Work out the finished part from the listing and answer in its coordinate system (mm). A direction names the side the tool comes from. Coordinates: 2 decimals unless noted, no trailing zeros. Loops run counter-clockwise (first coordinate to the right, second up) from the corner with the lowest first, then second, coordinate; pieces in that order, holes last. Notation, with made-up numbers: (17.5, 20.25) -> (61.5, 20.25) arc R9 ccw to (61.5, 29.25) -> close; hole circle Ø11 at (68, 60). An arc over 180 degrees is marked (long way). Use a Markdown table: item, result.
from build123d import *

# Parameters (mm, degrees)
EXTRUDE_1_DEPTH     = 2
SKETCH_2_R          = 1.6
CUT_EXTRUDE_1_DEPTH = 3
SKETCH_3_W          = 3
SKETCH_3_H          = 24
SKETCH_3_W_2        = 4
CUT_EXTRUDE_2_DEPTH = 3
SKETCH_4_W          = 10
SKETCH_4_H          = 2
EXTRUDE_2_DEPTH     = 2
SKETCH_5_R          = 0.5
CUT_EXTRUDE_3_DEPTH = 2
SKETCH_6_R          = 0.5
CUT_EXTRUDE_4_DEPTH = 2


with BuildPart() as part:
    # 草图1 → 凸台-拉伸1 (new body)
    with BuildSketch(Plane.XY):
        Polygon((0, 0), (17, 0), (17, 2.5), (20, 2.5), (20, 14.5), (17, 14.5), (17, 51.5), (0, 51.5), align=None)
    extrude(amount=EXTRUDE_1_DEPTH)

    # 草图2 → 切除-拉伸1 (cut, through all)
    with BuildSketch(Plane.XY.offset(2)):
        with Locations((9, 5.5)):
            Circle(SKETCH_2_R)
        with Locations((9, 16.5)):
            Circle(SKETCH_2_R)
    extrude(amount=-CUT_EXTRUDE_1_DEPTH, mode=Mode.SUBTRACT)

    # 草图3 → 切除-拉伸2 (cut, through all)
    with BuildSketch(Plane.XY.offset(2)):
        with Locations((15.5, 39.5)):
            Rectangle(SKETCH_3_W, SKETCH_3_H)
        with Locations((2, 39.5)):
            Rectangle(SKETCH_3_W_2, SKETCH_3_H)
    extrude(amount=-CUT_EXTRUDE_2_DEPTH, mode=Mode.SUBTRACT)

    # 草图4 → 凸台-拉伸2 (add)
    with BuildSketch(Plane(origin=(0, 51.5, 0), x_dir=(1, 0, 0), z_dir=(0, 1, 0))):
        with Locations((9, -1)):
            Rectangle(SKETCH_4_W, SKETCH_4_H)
    extrude(amount=EXTRUDE_2_DEPTH)

    # 草图5 → 切除-拉伸3 (cut)
    with BuildSketch(Plane(origin=(0, 0, 0), x_dir=(-1, 0, 0), z_dir=(0, 0, -1))):
        with Locations((-14, 27.5)):
            Circle(SKETCH_5_R)
        with Locations((-4, 27.5)):
            Circle(SKETCH_5_R)
    extrude(amount=-CUT_EXTRUDE_3_DEPTH, mode=Mode.SUBTRACT)

    # 草图6 → 切除-拉伸4 (cut)
    with BuildSketch(Plane(origin=(0, 0, 0), x_dir=(-1, 0, 0), z_dir=(0, 0, -1))):
        with Locations((-17, 14.5)):
            Circle(SKETCH_6_R)
        with Locations((-17, 2.5)):
            Circle(SKETCH_6_R)
    extrude(amount=-CUT_EXTRUDE_4_DEPTH, mode=Mode.SUBTRACT)


solid = part.part
Q1. Section B-B on y = 5.5 is taken. Determine the outline of the cut face in (x, z).
Solved:
| item | result |
|---|---|
| outline | (0, 0) -> (7.4, 0) -> (7.4, 2) -> (0, 2) -> close; (10.6, 0) -> (20, 0) -> (20, 2) -> (10.6, 2) -> close |
Q2. Given pin 1 Ø3.5 at (x, y) = (9, 5.5) entering from +Z; pin 2 Ø1 at (y, z) = (24, 1.5) entering from +X; pin 3 Ø0.6 at (x, z) = (1, 1) entering from +Y; pin 4 Ø1 at (y, z) = (39.5, 1) entering from +X, each flat-ended and moving along its own axis, determine where each tip first touches the part or whether it passes through.
Solved:
| item | result |
|---|---|
| pin 1 | z = 2 |
| pin 2 | x = 17 |
| pin 3 | y = 27.5 |
| pin 4 | x = 14 |
Q3. Section C-C on x = 2.25 is taken. Determine the outline of the cut face in (y, z).
Solved:
| item | result |
|---|---|
| outline | (0, 0) -> (27.5, 0) -> (27.5, 2) -> (0, 2) -> close |
Q4. Consider line 1 (Y direction, x = 9, z = 0.65); line 2 (X direction, y = 25.5, z = 0.1); line 3 (Y direction, x = 15.5, z = 1.35). Determine where each line is inside the solid, lowest interval first. Write a range as [from, to].
Solved:
| item | result |
|---|---|
| line 1 | [0, 3.9], [7.1, 14.9], [18.1, 53.5] |
| line 2 | [0, 17] |
| line 3 | [0, 27.5] |
Q5. Determine the mould class of faces 4 (the cylindrical face through (17, 14, 1)), 5 (the flat face through (14, 41, 1)), 6 (the flat face through (8, 0, 1)), 7 (the flat face through (0, 14, 1)) for opening direction X: pulls with the +X half, pulls with the -X half, needs draft (parallel to the pull), parting line crosses it, or undercut.
Solved:
| item | result |
|---|---|
| face 4 | undercut |
| face 5 | pulls with the +X half |
| face 6 | needs draft |
| face 7 | pulls with the -X half |
Q6. Section A-A on z = 1 is taken. Determine the outline of the cut face in (x, y), and give its area (3 significant figures).
Solved:
| item | result |
|---|---|
| outline | (0, 0) -> (17, 0) -> (17, 2) arc R0.5 cw (long way) to (17.5, 2.5) -> (20, 2.5) -> (20, 14.5) -> (17.5, 14.5) arc R0.5 cw (long way) to (17, 15) -> (17, 27.5) -> (14.5, 27.5) arc R0.5 cw (long way) to (14, 28) -> (14, 53.5) -> (4, 53.5) -> (4, 28) arc R0.5 cw (long way) to (3.5, 27.5) -> (0, 27.5) -> close; hole circle Ø3.2 at (9, 5.5); hole circle Ø3.2 at (9, 16.5) |
| area | 745 mm² |
Q7. Section D-D on y = 29 is taken. Determine the outline of the cut face in (x, z).
Solved:
| item | result |
|---|---|
| outline | (4, 0) -> (14, 0) -> (14, 2) -> (4, 2) -> close |
Q8. For faces 1 (the flat face through (16, 27.5, 1)), 2 (the flat face through (19, 2.5, 1)), 3 (the flat face through (2, 27.5, 1)), determine the directions among +Z, -Z, +X, -X, +Y, -Y from which every point of the face is accessible in a straight line to the end or side of a thin tool.
Solved:
| item | result |
|---|---|
| face 1 | +Z, -Z, +X, +Y |
| face 2 | +Z, -Z, +X, -Y |
| face 3 | +Z, -Z, -X, +Y |
